Model file for the job. Use its own axes, mm. Face numbers are marked on the shaded views. A direction names the side the tool comes from. Round coordinates to 2 decimals unless told otherwise and drop trailing zeros. Write each loop counter-clockwise with the first axis right and the second up, starting at its lowest first coordinate (ties: lowest second). Pieces come first, ordered by that corner, then holes. Notation, with made-up numbers: (38, 85.5) - (61, 85.5) arc R23 ccw to (61, 103.5) - close; hole circle Ø9 at (14, -10.5). An arc over 180 degrees is marked (long way). One line per item, written item: value.
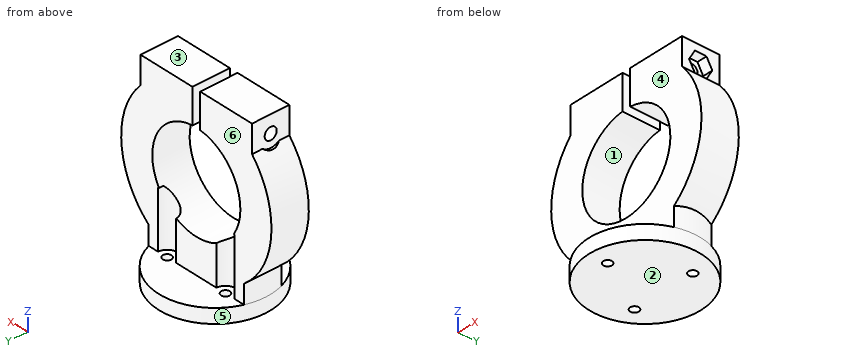
Autodesk Inventor part; units mm, degrees
ref_plane "YZ Plane" through (0, 0, 0) normal (1, 0, 0) x (0, 1, 0)
ref_plane "XZ Plane" through (0, 0, 0) normal (0, 1, 0) x (-1, 0, 0)
ref_plane "XY Plane" through (0, 0, 0) normal (0, 0, 1) x (1, 0, 0)
sketch "Skizze1" plane through (0, 0, 0) normal (0, 0, 1) x (1, 0, 0)
  circle A0 centre (-11.2583, 6.5) radius 1.5
  circle A1 centre (-11.2583, -6.5) radius 1.5
  circle A2 centre (0, -13) radius 1.5
  circle A3 centre (11.2583, -6.5) radius 1.5
  circle A4 centre (11.2583, 6.5) radius 1.5
  circle A5 centre (0, 13) radius 1.5
  arc A6 (14.3761, 1.8914) -> (11.9393, 3.5783) centre (12.3932, 1.6305) ccw
  arc A7 (14.3761, -1.8914) -> (14.3761, 1.8914) centre (0, 0) ccw
  arc A8 (11.9393, -3.5783) -> (14.3761, -1.8914) centre (12.3932, -1.6305) ccw
  arc A9 (11.9393, -3.5783) -> (9.0685, -8.5505) centre (11.2583, -6.5) ccw
  arc A10 (8.826, -11.5044) -> (9.0685, -8.5505) centre (7.6087, -9.9176) ccw
  arc A11 (5.5501, -13.3958) -> (8.826, -11.5044) centre (0, 0) ccw
  arc A12 (2.8707, -12.1288) -> (5.5501, -13.3958) centre (4.7846, -11.5481) ccw
  arc A13 (2.8707, -12.1288) -> (-2.8707, -12.1288) centre (0, -13) ccw
  arc A14 (-5.5501, -13.3958) -> (-2.8707, -12.1288) centre (-4.7846, -11.5481) ccw
  arc A15 (-8.826, -11.5044) -> (-5.5501, -13.3958) centre (0, 0) ccw
  arc A16 (-9.0685, -8.5505) -> (-8.826, -11.5044) centre (-7.6087, -9.9176) ccw
  arc A17 (-9.0685, -8.5505) -> (-11.9393, -3.5783) centre (-11.2583, -6.5) ccw
  arc A18 (-14.3761, -1.8914) -> (-11.9393, -3.5783) centre (-12.3932, -1.6305) ccw
  arc A19 (-14.3761, 1.8914) -> (-14.3761, -1.8914) centre (0, 0) ccw
  arc A20 (-11.9393, 3.5783) -> (-14.3761, 1.8914) centre (-12.3932, 1.6305) ccw
  arc A21 (-11.9393, 3.5783) -> (-9.0685, 8.5505) centre (-11.2583, 6.5) ccw
  arc A22 (-8.826, 11.5044) -> (-9.0685, 8.5505) centre (-7.6087, 9.9176) ccw
  arc A23 (-5.5501, 13.3958) -> (-8.826, 11.5044) centre (0, 0) ccw
  arc A24 (-2.8707, 12.1288) -> (-5.5501, 13.3958) centre (-4.7846, 11.5481) ccw
  arc A25 (-2.8707, 12.1288) -> (2.8707, 12.1288) centre (0, 13) ccw
  arc A26 (5.5501, 13.3958) -> (2.8707, 12.1288) centre (4.7846, 11.5481) ccw
  arc A27 (8.826, 11.5044) -> (5.5501, 13.3958) centre (0, 0) ccw
  arc A28 (9.0685, 8.5505) -> (8.826, 11.5044) centre (7.6087, 9.9176) ccw
  arc A29 (9.0685, 8.5505) -> (11.9393, 3.5783) centre (11.2583, 6.5) ccw
  circle A30 centre (0, 0) radius 17.5
  circle A31 centre (0, 0) radius 19.5
  point P0 (0, 0)
  dimension "d0" = 39
extrude "Extrusion1" add sketch "Skizze1" along normal blind 5 contours A7 A8 A9 A10 A11 A12 A13 A14 A15 A16 A17 A18 A19 A20 A21 A22 A23 A24 A25 A26 A27 A28 A29 A6 | A30 | A31
ref_plane "Arbeitsebene1" through (11.2583, -6.5, 0) normal (0, -1, 0) x (0, 0, 1)
sketch "Skizze7" plane through (11.2583, -6.5, 0) normal (0, -1, 0) x (0, 0, 1)
  line L0 (0, 21.0167) -> (5, 21.0167)
  line L1 (5, 21.0167) -> (5, 1.5)
  line L2 (5, 1.5) -> (0, 1.5)
  line L3 (0, 1.5) -> (0, 21.0167)
  line L4 (5, -7.1264) -> (0, -7.1264)
  line L5 (0, -7.1264) -> (0, -1.5)
  line L6 (0, -1.5) -> (5, -1.5)
  line L7 (5, -1.5) -> (5, -7.1264)
  line L8 (0, 29.6431) -> (5, 29.6431)
  line L9 (5, 29.6431) -> (5, 24.0167)
  line L10 (5, 24.0167) -> (0, 24.0167)
  line L11 (0, 24.0167) -> (0, 29.6431)
  line L12 (5, 1.5) -> (17, 1.5)
  line L13 (17, 1.5) -> (17, 21.0167)
  line L14 (17, 21.0167) -> (5, 21.0167)
  line L15 (5, 21.0167) -> (5, 1.5)
  arc A0 (50.9337, 12.7583) -> (50.9337, 9.7583) centre (34, 11.2583) ccw
  arc A1 (62.9612, 12.7583) -> (62.9612, 9.7583) centre (34, 11.2583) ccw
  line L16 (50.9337, 9.7583) -> (62.9612, 9.7583)
  line L17 (50.9337, 12.7583) -> (62.9612, 12.7583)
  line L18 (34, 11.2583) -> (5, 11.2583) construction
  line L19 (5, -7.1264) -> (11.5723, -7.1264)
  line L20 (5, 29.6431) -> (11.5723, 29.6431)
  line L21 (5, -7.1264) -> (5, 29.6431)
  point P0 (0, 11.2583)
  dimension "d26" = 3
  dimension "d27" = 17
  dimension "d28" = 12
extrude "Extrusion6" add sketch "Skizze7" against normal blind 13 contours L14 A1 L1 | L21 L9 L20 A1 L14 | A1 L12 L1 | A1 L14 L13 L12 | A1 L17 A0 L13 L14 | L12 A1 L19 L7 L21 | L12 L13 A0 L16 A1
sketch "Skizze8" plane through (1.5, -6.5, 50.9337) normal (-1, 0, 0) x (0, 0, 1)
  line L0 (12.0275, 0) -> (0, 0)
  line L1 (0, 0) -> (0, 13)
  line L2 (0, 13) -> (12.0275, 13)
  line L3 (12.0275, 13) -> (12.0275, 0)
  line L4 (-45.9337, 25.9422) -> (-45.9337, 19.5)
  line L5 (-45.9337, 19.5) -> (-45.9337, 13)
  line L6 (-45.9337, 13) -> (-33.8674, 13)
  line L7 (-33.8674, 13) -> (-33.8674, 0)
  line L8 (-33.8674, 0) -> (-45.9337, 0)
  line L9 (-45.9337, 0) -> (-45.9337, -6.5)
  line L10 (-45.9337, -6.5) -> (-50.9337, -6.5)
  line L11 (-50.9337, -6.5) -> (-50.9337, 19.5)
  line L12 (-50.9337, 19.5) -> (-50.9337, 25.9422)
  line L13 (-50.9337, 25.9422) -> (-45.9337, 25.9422)
  line L14 (-45.9337, 19.5) -> (-50.9337, 19.5)
  line L15 (-45.9337, -6.5) -> (-45.9337, -12.9422)
  line L16 (-45.9337, -12.9422) -> (-50.9337, -12.9422)
  line L17 (-50.9337, -12.9422) -> (-50.9337, -6.5)
  point P0 (-50.9337, 6.5)
extrude "Extrusion7" add sketch "Skizze8" against normal blind 20 contours L0 L1 L2 L3
sketch "Skizze9" plane through (-1.5, -6.5, 62.9612) normal (1, 0, 0) x (0, 0, -1)
  line L0 (12.0275, 0) -> (0, 0)
  line L1 (0, 0) -> (0, 13)
  line L2 (0, 13) -> (12.0275, 13)
  line L3 (12.0275, 13) -> (12.0275, 0)
  line L4 (57.9612, -12.9422) -> (57.9612, -6.5)
  line L5 (57.9612, -6.5) -> (57.9612, 0)
  line L6 (57.9612, 0) -> (45.8949, 0)
  line L7 (45.8949, 0) -> (45.8949, 13)
  line L8 (45.8949, 13) -> (57.9612, 13)
  line L9 (57.9612, 13) -> (57.9612, 19.5)
  line L10 (57.9612, 19.5) -> (62.9612, 19.5)
  line L11 (62.9612, 19.5) -> (62.9612, -6.5)
  line L12 (62.9612, -6.5) -> (62.9612, -12.9422)
  line L13 (62.9612, -12.9422) -> (57.9612, -12.9422)
  line L14 (57.9612, -6.5) -> (62.9612, -6.5)
  line L15 (57.9612, 19.5) -> (57.9612, 25.9422)
  line L16 (57.9612, 25.9422) -> (62.9612, 25.9422)
  line L17 (62.9612, 25.9422) -> (62.9612, 19.5)
  point P0 (62.9612, 6.5)
extrude "Extrusion8" add sketch "Skizze9" against normal blind 20 contours L0 L1 L2 L3
sketch "Skizze10" plane through (0, 0, 5) normal (0, 0, 1) x (1, 0, 0)
  circle A0 centre (0, 13) radius 1.5
  circle A1 centre (11.2583, 6.5) radius 1.5
  circle A2 centre (11.2583, -6.5) radius 1.5
  circle A3 centre (0, -13) radius 1.5
  circle A4 centre (-11.2583, -6.5) radius 1.5
  circle A5 centre (-11.2583, 6.5) radius 1.5
  circle A6 centre (0, 0) radius 19.5
  circle A7 centre (11.2583, 6.5) radius 3.5
  circle A8 centre (-11.2583, 6.5) radius 3.5
  line L0 (12.7583, 6.5) -> (9.7583, 6.5)
  point P0 (0, 0)
  dimension "d35" = 7
extrude "Extrusion9" cut sketch "Skizze10" along normal blind 20 contours L0 A1 | A1 L0 | A5 | A7 | A8
sketch "Skizze11" plane through (0, 0, 0) normal (0, 0, -1) x (-1, 0, 0)
  circle A0 centre (0, 13) radius 1.5
  circle A1 centre (-11.2583, 6.5) radius 1.5
  circle A2 centre (-11.2583, -6.5) radius 1.5
  circle A3 centre (0, -13) radius 1.5
  circle A4 centre (11.2583, -6.5) radius 1.5
  circle A5 centre (11.2583, 6.5) radius 1.5
  circle A6 centre (0, 0) radius 19.5
  point P0 (0, 0)
extrude "Extrusion10" add sketch "Skizze11" against normal up to surface (5 mm away) contours A0 | A2 | A4
sketch "Skizze13" plane through (-21.5, -6.5, 62.9612) normal (-1, 0, 0) x (0, 0, 1)
  line L0 (-12.0275, 0) -> (0, 0)
  line L1 (-12.0275, 0) -> (-12.0275, 13)
  line L2 (0, 13) -> (-12.0275, 13)
  line L3 (0, 0) -> (0, 13)
  line L4 (-12.0275, 0) -> (0, 0)
  line L5 (0, 0) -> (0, 13)
  line L6 (0, 13) -> (-12.0275, 13)
  line L7 (-12.0275, 13) -> (-12.0275, 0)
  line L8 (-12.0275, 0) -> (0, 13) construction
  line L9 (0, 0) -> (-12.0275, 13) construction
  point P0 (-62.9612, 6.5)
  point P1 (-6.0137, 6.5)
hole "Bohrung2" at (-21.5, 0, 56.9474) direction (1, 0, 0) diameter 4.2 end through all
sketch "Skizze14" plane through (-21.5, -6.5, 62.9612) normal (-1, 0, 0) x (0, 0, 1)
  circle A0 centre (-6.0137, 6.5) radius 2.1
  line L0 (-9.4997, 0) -> (-9.4997, 13)
  line L1 (-9.4997, 0) -> (0, 0)
  line L2 (0, 0) -> (0, 13)
  line L3 (0, 13) -> (-9.4997, 13)
  circle A1 centre (-6.0137, 6.5) radius 4.5
  point P0 (-62.9612, 6.5)
  dimension "d47" = 9
extrude "Extrusion11" cut sketch "Skizze14" along normal blind 2 contours A0 | A1 L0 | L0 A1
sketch "Skizze15" plane through (21.5, -6.5, 50.9337) normal (1, 0, 0) x (0, 0, -1)
  circle A0 centre (-6.0137, 6.5) radius 2.1
  line L0 (-2.5278, 13) -> (-2.5278, 0)
  line L1 (-2.5278, 13) -> (-12.0275, 13)
  line L2 (-12.0275, 13) -> (-12.0275, 0)
  line L3 (-12.0275, 0) -> (-2.5278, 0)
  line L4 (-6.0137, 10.5415) -> (-2.5137, 8.5207)
  line L5 (-2.5137, 8.5207) -> (-2.5137, 4.4793)
  line L6 (-2.5137, 4.4793) -> (-6.0137, 2.4585)
  line L7 (-6.0137, 2.4585) -> (-9.5137, 4.4793)
  line L8 (-9.5137, 4.4793) -> (-9.5137, 8.5207)
  line L9 (-9.5137, 8.5207) -> (-6.0137, 10.5415)
  line L10 (-12.0275, 13) -> (-12.0275, 0)
  point P0 (50.9337, 6.5)
  dimension "d50" = 7
extrude "Extrusion12" cut sketch "Skizze15" along normal mid plane 7 contours A0 | L4 L5 L6 L0 | L0 L6 L7 L8 L9 L4
sketch "Skizze16" plane through (0, 0, 5) normal (0, 0, 1) x (1, 0, 0)
  line L0 (-18.3848, -6.5) -> (-18.3848, 6.5)
  arc A0 (-18.3848, 6.5) -> (-18.3848, -6.5) centre (0, 0) ccw
  line L1 (18.3848, 6.5) -> (18.3848, -6.5)
  arc A1 (18.3848, -6.5) -> (18.3848, 6.5) centre (0, 0) ccw
  point P0 (0, 0)
extrude "Extrusion13" add sketch "Skizze16" along normal blind 10
sketch "Skizze2" plane through (0, 0, 5) normal (0, 0, 1) x (1, 0, 0)
  circle A0 centre (0, 0) radius 7.5
  dimension "d3" = 15
  dimension "d20" = 7
  dimension "d8" = 7
sketch "Skizze4" plane through (0, 0, 10) normal (0, 0, 1) x (1, 0, 0)
  point P0 (0, 0)
sketch "Skizze5" plane through (0, 0, 3) normal (0, 0, -1) x (-1, 0, 0)
  circle A0 centre (0, 0) radius 2
  circle A1 centre (0, 0) radius 2
properties part number "GripperMountProxxon" material "ABS-Kunststoff"
1. Mould opens along Z. For the marked faces 1, 2 and 3 say: released by +Z, released by -Z, zero draft, split by the parting line, or undercut.
Report:
face 1: undercut
face 2: released by -Z
face 3: released by +Z
2. Band-saw the part on D-D on z = 46. Write the cut outline in (x, y).
Report:
outline: (-26.4, -6.5) - (-12.04, -6.5) - (-12.04, 6.5) - (-26.4, 6.5) - close; (12.04, -6.5) - (26.4, -6.5) - (26.4, 6.5) - (12.04, 6.5) - close
3. Band-saw the part on B-B on z = 34. Write the cut outline in (x, y).
Report:
outline: (-29, -6.5) - (-17, -6.5) - (-17, 6.5) - (-29, 6.5) - close; (17, -6.5) - (29, -6.5) - (29, 6.5) - (17, 6.5) - close
4. Band-saw the part on A-A on y = 0. Write the cut outline in (x, z), plus the area to 3 significant figures.
Report:
outline: (-22.38, 52.45) arc R29 ccw to (-19.5, 12.53) - (-19.5, 0) - (19.5, 0) - (19.5, 12.53) arc R29 ccw to (21.51, 53.45) - (18, 53.45) - (18, 54.85) - (1.5, 54.85) - (1.5, 50.93) arc R17 cw (long way) to (-1.5, 50.93) - (-1.5, 54.85) - (-21.5, 54.85) - (-21.5, 52.45) - close; (-21.5, 59.05) - (-1.5, 59.05) - (-1.5, 62.96) - (-21.5, 62.96) - close; (1.5, 59.05) - (18, 59.05) - (18, 60.45) - (21.5, 60.45) - (21.5, 62.96) - (1.5, 62.96) - close
area: 1,930 mm²
5. Tool access for the marked faces 4, 5 and 6: list every direction of +Z, -Z, +X, -X, +Y, -Y with a clear straight run to the whole face (end or side of a thin tool).
Report:
face 4: +Z, +X, -X, -Y
face 5: -Z
face 6: +Z, +X, -X, +Y
6. Band-saw the part on C-C on x = 5. Write the cut outline in (y, z).
Report:
outline: (-18.85, 0) - (18.85, 0) - (18.85, 5) - (6.5, 5) - (6.5, 17.75) - (-6.5, 17.75) - (-6.5, 5) - (-18.85, 5) - close; (-6.5, 50.25) - (6.5, 50.25) - (6.5, 62.96) - (-6.5, 62.96) - close; hole circle Ø4.2 at (0, 56.95)
7. Wall check: probe 1 along X at (y, z) = (6.5, 2.85); probe 2 along X at (y, z) = (2, 34); probe 3 along Y at (x, z) = (0, 1.2). Give the ranges that are in metal, low to high. Write a range as [from, to].
Report:
probe 1: [-18.38, -12.76], [-9.76, 9.76], [12.76, 18.38]
probe 2: [-29, -17], [17, 29]
probe 3: [-19.5, -14.5], [-11.5, 19.5]
8. Drop flat-ended pins along their axis: pin 1 (4 mm diameter, centred on x = -1.5, z = 11.5, fed in from +Y); pin 2 (4 mm diameter, centred on x = 3, z = 18, fed in from -Y); pin 3 (8.5 mm diameter, centred on y = 2.5, z = 58, fed in from -X); pin 4 (4 mm diameter, centred on x = -13.5, z = 29.5, fed in from -Y). Give the stop position or say it passes through.
Report:
pin 1: y = 6.5
pin 2: y = -6.5
pin 3: x = -21.5
pin 4: through
